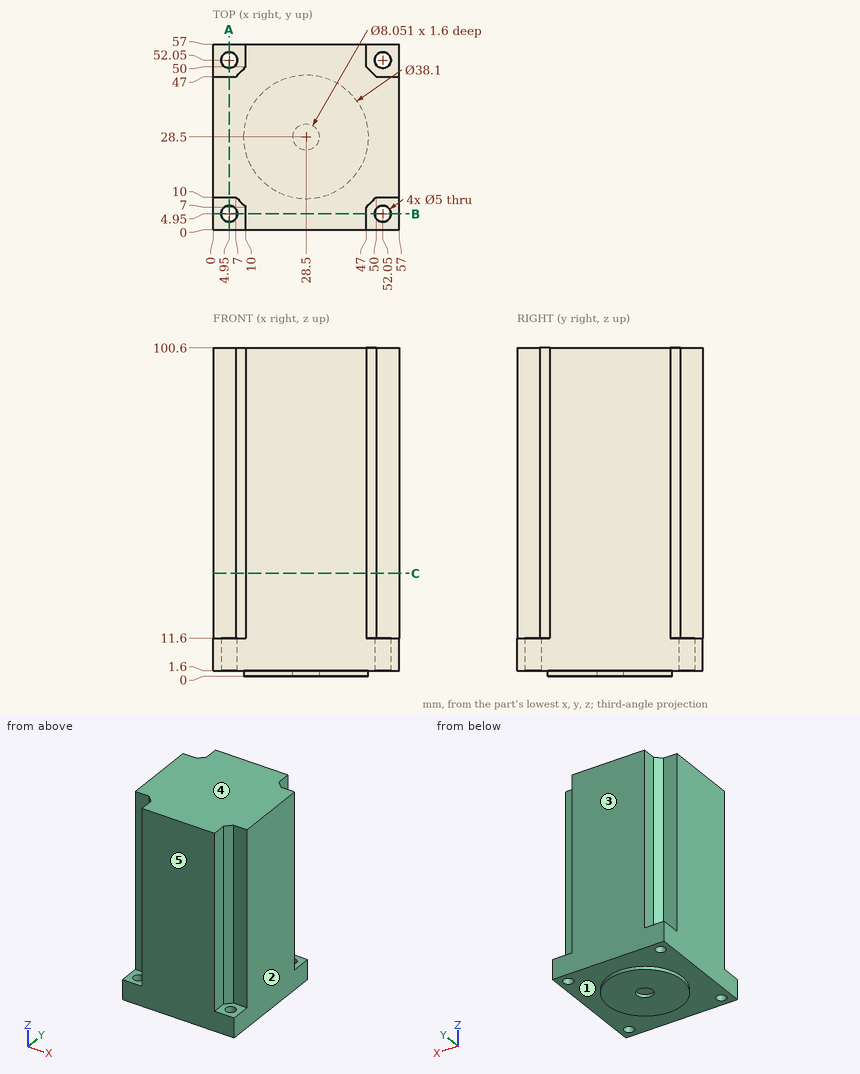
Study the drawing (mm; zero at the part's minimum x, y, z) and answer. A direction names the side the tool comes from. Coordinates: 2 decimals unless noted, no trailing zeros. Loops run counter-clockwise (first coordinate to the right, second up) from the corner with the lowest first, then second, coordinate; pieces in that order, holes last. Notation, with made-up numbers: M 20.5,36.25 L 73.5,36.25 A22 ccw 73.5,64.25 Z; hole C 61,57.5 d5. An arc over 180 degrees is marked long. Answer as a JSON object with one key per item and string values. Group by question number.
Item 1: Each of these flat-tipped pins is pushed along its axis until it touches: P1, Ø6, axis at x = 52.05, y = 52.05, coming from the +Z side; P2, Ø5, axis at x = 48.5, z = 51.5, coming from the -Y side; P3, Ø3.5, axis at y = 53.5, z = 49, coming from the -X side; P4, Ø4, axis at x = 4.95, y = 4.95, coming from the +Z side. Where does it stop, or does it pass through?
Item 2: Determine the mould class of the marked faces 3, 4 and 5 for opening direction Y: +Y half, -Y half, draft (parallel to the pull), parting line (faces both ways), or undercut.
Item 3: Section A-A (x = 4.95) is taken. Write down the section's boundary in (y, z).
Item 4: Consider L1, parallel to Y at x = 52, z = 8; L2, parallel to X at y = 4, z = 6. Determine where each line is inside the solid, lowest interval first.
Item 5: Which of the six approach directions +Z, -Z, +X, -X, +Y, -Y give full straight-line access (tool end or side, diameter ignored) to the marked faces 1 and 2?
Item 6: Section C-C (z = 31.5) is taken. Write down the section's boundary in (x, y), and give its area (3 significant figures).
Solved:
{
 "1": {"P1": "stops at z = 11.6", "P2": "stops at y = 0", "P3": "stops at x = 10", "P4": "passes through"},
 "2": {"face 3": "+Y half", "face 4": "draft", "face 5": "-Y half"},
 "3": {"outline": "M 0,1.6 L 2.45,1.6 L 2.45,11.6 L 0,11.6 Z; M 7.45,1.6 L 49.55,1.6 L 49.55,11.6 L 47,11.6 L 47,100.6 L 10,100.6 L 10,11.6 L 7.45,11.6 Z; M 54.55,1.6 L 57,1.6 L 57,11.6 L 54.55,11.6 Z"},
 "4": {"L1": "y = 0 to 2.45, 7.45 to 49.55, 54.55 to 57", "L2": "x = 0 to 2.64, 7.26 to 49.74, 54.36 to 57"},
 "5": {"face 1": "-Z", "face 2": "+Z, -Z, +X, +Y, -Y"},
 "6": {"outline": "M 0,10 L 7,10 L 10,7 L 10,0 L 47,0 L 47,7 L 50,10 L 57,10 L 57,47 L 50,47 L 47,50 L 47,57 L 10,57 L 10,50 L 7,47 L 0,47 Z", "area": "2,870 mm2"}
}
